from build123d import *

# Parameters (mm, degrees)
F3_DEPTH = 5.842
F1_E1_W  = 68.4977713972
F1_E1_H  = 25.4
F4_DEPTH = 55.626


with BuildPart() as f3:
    # F2 (on Top) → F3 (new body)
    with BuildSketch(Plane.XY):
        Polygon((-66.1953240633, 37.8464572132), (-66.1953240633, 32.953761518), (-66.1953240633, -46.768438071), (51.8050417304, -46.768438071), (58.4245696664, -46.768438071), (58.4245696664, 37.8464572132), align=None)
    extrude(amount=F3_DEPTH)

    # F1_E1 (on explicit) → F4 (join)
    with BuildSketch(Plane(origin=(-37.4147482216, -32.3781482875, 0), x_dir=(1, 0, 0), z_dir=(0, -1, 0))):
        with Locations((34.2488856986, 12.7)):
            Rectangle(F1_E1_W, F1_E1_H)
    extrude(amount=-F4_DEPTH)


solid = f3.part
Could you check a few things on this model? Use its own coordinates, in mm. A direction names the side the tool comes from. Give positions to 0.01 mm unless a question says otherwise; leave off trailing zeros. Write each loop counter-clockwise with the first axis right and the second up, starting at its lowest first coordinate (ties: lowest second). Pieces come first, ordered by that corner, then holes. Notation, with made-up numbers: (88.5, 44) -> (93.5, 44) arc R28 cw to (93.5, 78) -> close; hole circle Ø7 at (83.5, 85). An arc over 180 degrees is marked (long way). Answer as CSV lines item,"result". Start each with the question number.
(1) I'm going to push flat-ended pins straight in: pin 1 Ø10 at (x, y) = (37.5, 13.5) entering from +Z; pin 2 Ø5 at (x, y) = (18.5, -34) entering from +Z; pin 3 Ø10 at (x, z) = (-19, 16.5) entering from +Y; pin 4 Ø1 at (y, z) = (22, 10) entering from +X. Where does each tip first touch, or does it pass through?
(2) If we section it at B-B, the plane x = -17: Write out the boundary of the cut face in (y, z), and give its area (3 significant figures).
(3) Which directions (+Z, -Z, +X, -X, +Y, -Y) give clear straight access to the entire face, cutting with the end or side of a thin tool? Please do faces 1 (the face through (-4, -32.378, 16)), 2 (the face through (-4, 23.248, 16)), 3 (the face through (-37.415, -5, 15)).
(4) If we section it at D-D, the plane y = 31.5: Write out the boundary of the cut face in (x, z).
(5) If we section it at C-C, the plane z = 14.75: Write out the boundary of the cut face in (x, y).
(6) If we section it at A-A, the plane y = -2: Write out the boundary of the cut face in (x, z).
(7) Please list where these lines run through material, in increasing order: line 1 (Y direction, x = 16, z = 23.25); line 2 (Z direction, x = -45, y = 4); line 3 (X direction, y = -7.5, z = 16.5).
Answer list:
1,pin 1,"z = 5.84"
1,pin 2,"z = 25.4"
1,pin 3,"y = 23.25"
1,pin 4,"x = 31.08"
2,outline,"(-46.77, 0) -> (37.85, 0) -> (37.85, 5.84) -> (23.25, 5.84) -> (23.25, 25.4) -> (-32.38, 25.4) -> (-32.38, 5.84) -> (-46.77, 5.84) -> close"
2,area,"1,580 mm^2"
3,face 1,"+Z, +X, -X, -Y"
3,face 2,"+Z, +X, -X, +Y"
3,face 3,"+Z, -X, +Y, -Y"
4,outline,"(-66.2, 0) -> (58.42, 0) -> (58.42, 5.84) -> (-66.2, 5.84) -> close"
5,outline,"(-37.41, -32.38) -> (31.08, -32.38) -> (31.08, 23.25) -> (-37.41, 23.25) -> close"
6,outline,"(-66.2, 0) -> (58.42, 0) -> (58.42, 5.84) -> (31.08, 5.84) -> (31.08, 25.4) -> (-37.41, 25.4) -> (-37.41, 5.84) -> (-66.2, 5.84) -> close"
7,line 1,"-32.38 to 23.25"
7,line 2,"0 to 5.84"
7,line 3,"-37.41 to 31.08"
